Autodesk Inventor part; units mm, degrees
ref_plane "YZ Plane" through (0, 0, 0) normal (1, 0, 0) x (0, 1, 0)
ref_plane "XZ Plane" through (0, 0, 0) normal (0, 1, 0) x (-1, 0, 0)
ref_plane "XY Plane" through (0, 0, 0) normal (0, 0, 1) x (1, 0, 0)
sketch "Sketch1" plane through (0, 0, 0) normal (0, 1, 0) x (-1, 0, 0)
  line L0 (0, 3.2476) -> (0, -3.2476)
  line L1 (0, -3.2476) -> (-1.25, -3.2476)
  line L2 (-1.25, -3.2476) -> (-1.5, -2.9976)
  line L3 (-1.5, -2.9976) -> (-1.5, 2.6524)
  line L4 (-1.6, 2.7524) -> (-2.85, 2.7524)
  line L5 (-2.85, 2.7524) -> (-2.85, 3.0024)
  line L6 (0, 3.2476) -> (-1.1547, 4.4024)
  line L7 (-1.1547, 4.4024) -> (-1.5, 4.4024)
  arc A0 (-1.5, 4.4024) -> (-2.85, 3.0024) centre (0, 1.605) ccw
  line L8 (-1.1547, 4.4024) -> (-0.5774, 5.4024) construction
  line L9 (-0.5774, 5.4024) -> (0.5774, 5.4024) construction
  line L10 (0.5774, 5.4024) -> (1.1547, 4.4024) construction
  line L11 (1.1547, 4.4024) -> (0.5774, 3.4024) construction
  line L12 (0.5774, 3.4024) -> (-0.5774, 3.4024) construction
  line L13 (-0.5774, 3.4024) -> (-1.1547, 4.4024) construction
  arc A1 (-1.5, 2.6524) -> (-1.6, 2.7524) centre (-1.6, 2.6524) ccw
  point P0 (0, 0)
  point P1 (-1.5, 2.7524)
  point P2 (0, 0)
  point P3 (0, 4.4024)
  dimension "d0" = 3
  dimension "d1" = 6
  dimension "d2" = 0.25
  dimension "d3" = 135
  dimension "d4" = 5.7
  dimension "d5" = 3
  dimension "d6" = 1.65
  dimension "d7" = 2
  dimension "d8" = 0.25
  dimension "d15" = 3.2
revolve "Revolution1" add sketch "Sketch1" angle 360 about axis through (0, 0, 3.2476) along (0, 0, -1)
sketch "Sketch2" plane through (0, 0, 4.4024) normal (0, 0, 1) x (1, 0, 0)
  circle A0 centre (0, 0) radius 1.1547
  circle A1 centre (0, 0) radius 1.5
  line L0 (-1.1547, 0) -> (-0.5774, 1)
  line L1 (-0.5774, 1) -> (0.5774, 1)
  line L2 (0.5774, 1) -> (1.1547, 0)
  line L3 (1.1547, 0) -> (0.5774, -1)
  line L4 (0.5774, -1) -> (-0.5774, -1)
  line L5 (-0.5774, -1) -> (-1.1547, 0)
  point P0 (0, 0)
extrude "Extrusion1" cut sketch "Sketch2" against normal blind 1.2 contours L3 L4 L5 L0 L1 L2
thread "Thread1"
properties part number "Bolt_M3x0.35_6mm_BH" material "Stainless Steel"
For this review, take the finished solid that the model builds, in its own axes (mm). A direction names the side the tool comes from. Round coordinates to 2 decimals unless told otherwise and drop trailing zeros. Write each loop counter-clockwise with the first axis right and the second up, starting at its lowest first coordinate (ties: lowest second). Pieces come first, ordered by that corner, then holes. Notation, with made-up numbers: M -39.75,19 L -8.75,19 A24 ccw -8.75,52 Z; hole C -26.5,-31.5 d6. An arc over 180 degrees is marked long. One line per item, written item: value. Start each with the question number.
(1) Machinability: for faces 1 (the flat face through (0, 0, 3.202)), 2 (the flat face through (0, 0, -3.248)), which of the approach directions +Z, -Z, +X, -X, +Y, -Y give a long, thin tool a straight path to every point of the face, cutting with its end or side? Answer none if there is none.
(2) Wall thickness on line 1 (Y direction, x = 0, z = -0.75); line 2 (Z direction, x = -0.4, y = -0.7); line 3 (X direction, y = -0.3, z = 3.25): over which ranges is each line inside the solid? List them lowest first.
(3) The part is to be moulded in two halves that separate along Y. For faces 3 (the flat face through (0, 2, 2.752)), 4 (the cylindrical face through (-1.5, 0.07, -0.13)), 5 (the flat face through (-0.86, -0.51, 3.81)), say which applies: released by +Y, released by -Y, zero draft, split by the parting line, or undercut.
(4) We need section A-A (z = -1.25). Give the boundary of the cut face in (x, y), and give its area (3 significant figures).
(5) Insertion check: pin 1 (3 mm diameter, centred on x = 1, z = 1, fed in from +Y); pin 2 (1.5 mm diameter, centred on y = -2, z = -1.5, fed in from +X); pin 3 (3 mm diameter, centred on y = 1, z = 3.5, fed in from +X); pin 4 (0.6 mm diameter, centred on x = 0, y = 0, fed in from +Z). Each pin has a flat end and moves straight along its axis. Give the tip position at first contact, or say it passes through.
Result:
1. face 1: +Z
1. face 2: -Z, +X, -X, +Y, -Y
2. line 1: -1.5 to 1.5
2. line 2: -3.25 to 3.2
2. line 3: -2.7 to -0.98, 0.98 to 2.7
3. face 3: zero draft
3. face 4: split by the parting line
3. face 5: undercut
4. outline: C 0,0 d3
4. area: 7.07 mm²
5. pin 1: y = 1.5
5. pin 2: x = 0.83
5. pin 3: x = 2.85
5. pin 4: z = 3.2
